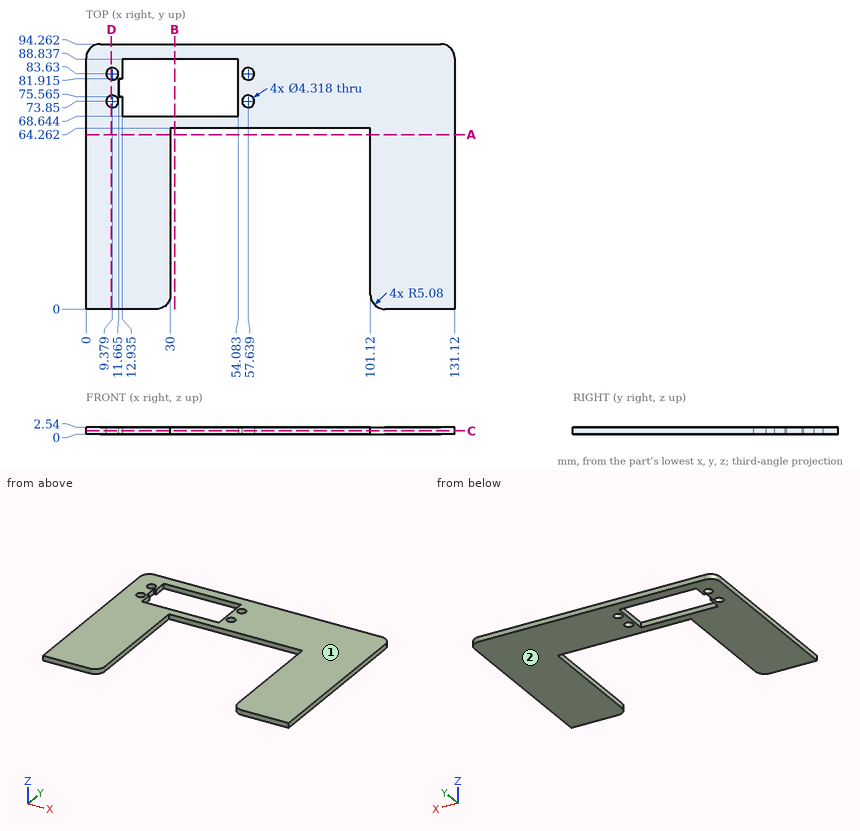
Print and shaded views of the part. All mm, measured from the part's lowest x, y and z. Coordinates: 2 decimals unless noted, no trailing zeros. Order: outer loops, then holes, each group sorted by start corner. A loop starts at its lowest first (then second) coordinate and runs counter-clockwise, first axis right, second up. Notation, with made-up numbers: (73.5, 72) - (129.5, 72) arc R29 ccw to (129.5, 100) - close; hole circle Ø8 at (-3, 67.25). An arc over 180 degrees is marked (long way). Put each result on its own line as item: value.
1. Pull direction Z, two halves, no side cores. Call the marked faces 1 and 2: pulls with the +Z half, pulls with the -Z half, needs draft (parallel to the pull), parting line crosses it, or undercut.
Answer sheet:
face 1: pulls with the +Z half
face 2: pulls with the -Z half
2. Saw through at B-B (x = 31.5). Write the cut outline in (y, z), and give its area (3 significant figures).
Answer sheet:
outline: (64.26, 0) - (68.64, 0) - (68.64, 2.54) - (64.26, 2.54) - close; (88.84, 0) - (94.26, 0) - (94.26, 2.54) - (88.84, 2.54) - close
area: 24.9 mm^2
3. Saw through at C-C (z = 1.2). Give the number of separate pieces and of enclosed holes in the cut face, and give its area (3 significant figures).
Answer sheet:
separate pieces: 1
enclosed holes: 5
area: 6,870 mm^2
4. Probe line 1 along X through (y, z) = (34, 0.3); line 2 along X through (y, z) = (84, 2.35) (1 decimal); line 3 along Y through (x, z) = (25, 1.4). List the from-to ranges inside material, lowest first. Write a range as [from, to].
Answer sheet:
line 1: x = [0, 30], [101.12, 131.12]
line 2: x = [0, 7.3], [11.5, 12.9], [54.1, 55.5], [59.8, 131.1]
line 3: y = [0, 68.64], [88.84, 94.26]
5. Saw through at D-D (x = 9). Write the cut outline in (y, z) (1 decimal).
Answer sheet:
outline: (0, 0) - (71.7, 0) - (71.7, 2.5) - (0, 2.5) - close; (76, 0) - (81.5, 0) - (81.5, 2.5) - (76, 2.5) - close; (85.8, 0) - (94.3, 0) - (94.3, 2.5) - (85.8, 2.5) - close
6. Saw through at A-A (y = 62). Write the cut outline in (x, z).
Answer sheet:
outline: (0, 0) - (30, 0) - (30, 2.54) - (0, 2.54) - close; (101.12, 0) - (131.12, 0) - (131.12, 2.54) - (101.12, 2.54) - close
7. Drop flat-ended pins along their axis: P1, Ø0.8, axis at x = 25.5, z = 1, coming from the -Y side; P2, Ø1, axis at x = 103.5, z = 1.5, coming from the -Y side. Give the stop position or say it passes through.
Answer sheet:
P1: stops at y = 0
P2: stops at y = 0.5
